The model under review builds one solid part; all positions refer to its coordinate system, in mm. Round coordinates to 2 decimals unless told otherwise and drop trailing zeros. Write each loop counter-clockwise with the first axis right and the second up, starting at its lowest first coordinate (ties: lowest second). Pieces come first, ordered by that corner, then holes.
Item 1: To check wall thickness, follow L1, parallel to X at y = 6, z = 2.5; L2, parallel to X at y = 22, z = 29; L3, parallel to Y at x = 413.5, z = 19. State the ranges of each line that lie inside material, in increasing order.
Item 2: Clearance check with flat-ended pins moving along their axes: pin 1 Ø5 at (y, z) = (-11, 31) entering from -X; pin 2 Ø1.5 at (y, z) = (17, 27) entering from -X; pin 3 Ø1 at (y, z) = (0, 13.5) entering from -X. State where each tip first meets the part, or that it passes through.
Item 3: Add section A-A (y = 9.5). Give the boundary of the cut face in (x, z), plus the area to 3 significant figures.
Item 4: Add section B-B (z = 35). Give the boundary of the cut face in (x, y), plus the area to 3 significant figures.
```python
from build123d import *

# Parameters (mm, degrees)
SALIENTE_EXTRUIR1_DEPTH      = 50.8
SALIENTE_EXTRUIR1_DEPTH_BACK = 1
CROQUIS1_W                   = 914.4
CROQUIS1_H                   = 50.8
CORTAR_EXTRUIR2_DEPTH        = 461.825606927
CORTAR_EXTRUIR3_DEPTH        = 461.825606927
CORTAR_EXTRUIR4_DEPTH        = 461.825606927


with BuildPart() as part:
    # Croquis1 → Saliente-Extruir1 (new, two sides: drawn at the far end of the back side and taken through both)
    with BuildSketch(Plane.XY.offset(-SALIENTE_EXTRUIR1_DEPTH_BACK)):
        Rectangle(CROQUIS1_W, CROQUIS1_H)
    extrude(amount=SALIENTE_EXTRUIR1_DEPTH + SALIENTE_EXTRUIR1_DEPTH_BACK)

    # Croquis3 → Cortar-Extruir2 (cut, through all)
    with BuildSketch(Plane.XY.offset(50.8)):
        Polygon((-437.2, 25.4), (-457.2, 25.4), (-457.2, -25.4), align=None)
    extrude(amount=-CORTAR_EXTRUIR2_DEPTH, mode=Mode.SUBTRACT)

    # Croquis4 → Cortar-Extruir3 (cut, through all)
    with BuildSketch(Plane(origin=(0, 0, -1), x_dir=(-1, 0, 0), z_dir=(0, 0, -1))):
        Polygon((-437.2, 25.4), (-457.2, 25.4), (-457.2, -25.4), align=None)
    extrude(amount=-CORTAR_EXTRUIR3_DEPTH, mode=Mode.SUBTRACT)

    # Croquis6 → Cortar-Extruir4 (cut, through all)
    with BuildSketch(Plane.XY.offset(50.8)):
        Polygon((-437.2, 25.4), (-457.2, -25.4), (-406.4, 25.4), align=None)
        Polygon((437.2, 25.4), (406.4, 25.4), (457.2, -25.4), align=None)
    extrude(amount=-CORTAR_EXTRUIR4_DEPTH, mode=Mode.SUBTRACT)


solid = part.part
```
Numbers:
1. L1: x = -425.8 to 425.8
1. L2: x = -409.8 to 409.8
1. L3: y = -25.4 to 18.3
2. pin 1: stops at x = -445.3
2. pin 2: stops at x = -415.55
2. pin 3: stops at x = -432.3
3. outline: (-422.3, -1) - (422.3, -1) - (422.3, 50.8) - (-422.3, 50.8) - close
3. area: 43,800 mm2
4. outline: (-457.2, -25.4) - (457.2, -25.4) - (406.4, 25.4) - (-406.4, 25.4) - close
4. area: 43,900 mm2
